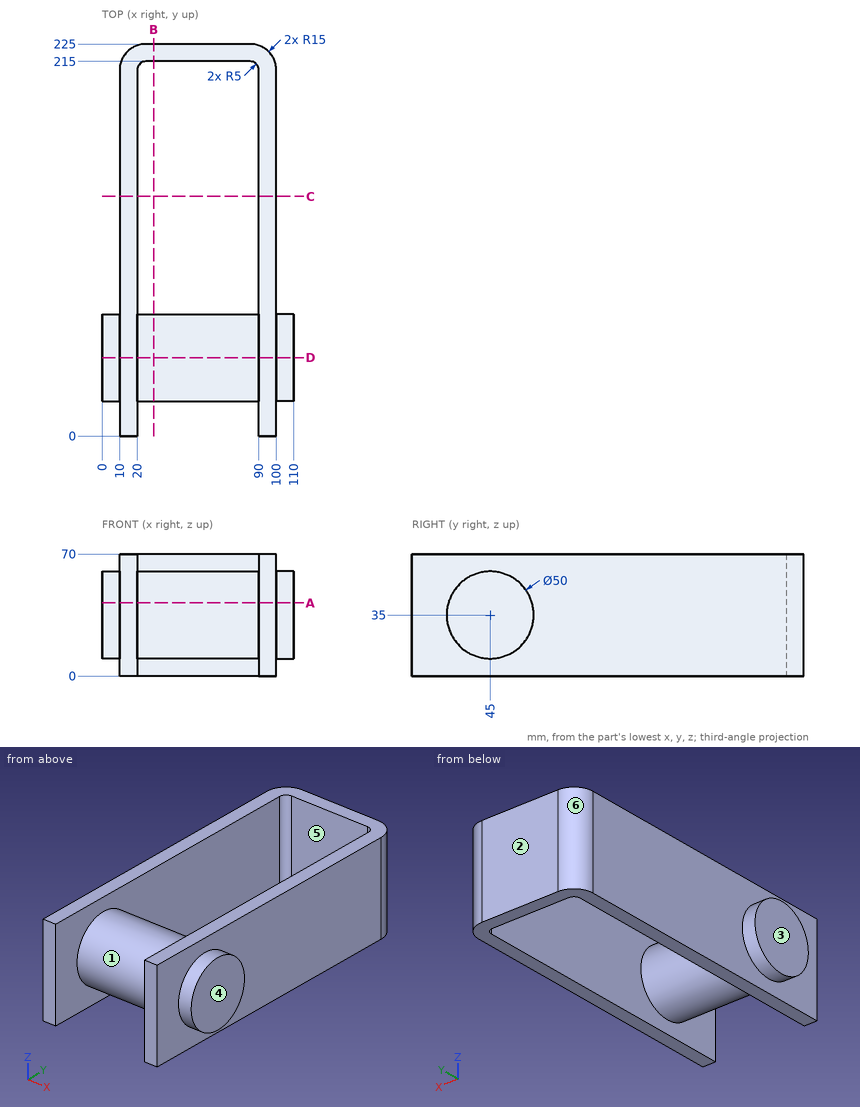
Study the drawing (mm; zero at the part's minimum x, y, z) and answer. A direction names the side the tool comes from. Round coordinates to 2 decimals unless told otherwise and drop trailing zeros. Write each loop counter-clockwise with the first axis right and the second up, starting at its lowest first coordinate (ties: lowest second). Pieces come first, ordered by that corner, then holes.
1) A cutting plane is placed at A-A (z = 42). Give the vertices of the cut face in (x, y).
2) Given pin 1 Ø21 at (y, z) = (82.5, 51) entering from -X; pin 2 Ø6 at (y, z) = (65.5, 34.5) entering from -X; pin 3 Ø6 at (y, z) = (149, 37) entering from +X; pin 4 Ø6 at (x, z) = (56, 39) entering from -Y, each flat-ended and moving along its own axis, determine where each tip first touches the part or whether it passes through.
3) The mould has two halves that part along X. Classify the marked faces 1, 2, 3 and 4: pulls with the +X half, pulls with the -X half, needs draft (parallel to the pull), parting line crosses it, or undercut.
4) A cutting plane is placed at B-B (x = 29.5). Give the vertices of the cut face in (y, z).
5) A cutting plane is placed at D-D (y = 45). Give the vertices of the cut face in (x, z), plus the area to 3 significant figures.
6) A cutting plane is placed at C-C (y = 137.5). Give the vertices of the cut face in (x, z).
7) Straight lines are drawn through the part: line 1 (X direction, y = 151, z = 53.5); line 2 (Y direction, x = 29, z = 40.5); line 3 (Y direction, x = 24, z = 44). For each, find the intervals that lie inside material, in ascending order.
8) A tool of negligible diameter and unlimited length cuts with its end or side. For the marked faces 5 and 6, from which of +Z, -Z, +X, -X, +Y, -Y can it reach the whole face along a straight path? Write none if from no direction.
Completed:
1. outline: (0, 21) - (10, 21) - (10, 0) - (20, 0) - (20, 21) - (90, 21) - (90, 0) - (100, 0) - (100, 21) - (110, 21) - (110, 69) - (100, 69) - (100, 210) arc R15 ccw to (85, 225) - (25, 225) arc R15 ccw to (10, 210) - (10, 69) - (0, 69) - close; hole (20, 69) - (90, 69) - (90, 210) arc R5 ccw to (85, 215) - (25, 215) arc R5 ccw to (20, 210) - close
2. pin 1: stops at x = 10
2. pin 2: stops at x = 0
2. pin 3: stops at x = 100
2. pin 4: stops at y = 20.02
3. face 1: undercut
3. face 2: needs draft
3. face 3: pulls with the -X half
3. face 4: pulls with the +X half
4. outline: circle Ø50 at (45, 35); (215, 0) - (225, 0) - (225, 70) - (215, 70) - close
5. outline: (0, 10) - (10, 10) - (10, 0) - (20, 0) - (20, 10) - (90, 10) - (90, 0) - (100, 0) - (100, 10) - (110, 10) - (110, 60) - (100, 60) - (100, 70) - (90, 70) - (90, 60) - (20, 60) - (20, 70) - (10, 70) - (10, 60) - (0, 60) - close
5. area: 5,900 mm2
6. outline: (10, 0) - (20, 0) - (20, 70) - (10, 70) - close; (90, 0) - (100, 0) - (100, 70) - (90, 70) - close
7. line 1: x = 10 to 20, 90 to 100
7. line 2: y = 20.61 to 69.39, 215 to 225
7. line 3: y = 21.68 to 68.32, 214.9 to 224.97
8. face 5: +Z, -Z
8. face 6: +Z, -Z, -X, +Y
